The listing builds one solid part. Answer for the finished solid, in the listing's coordinates (mm). Give positions to 0.01 mm unless a question says otherwise; leave off trailing zeros. Order: outer loops, then holes, each group sorted by start corner. A loop starts at its lowest first (then second) coordinate and runs counter-clockwise, first axis right, second up. Notation, with made-up numbers: (-18, 13.25) - (11, 13.25) arc R26 cw to (11, 44.25) - close; hole circle Ø3 at (37.25, 82.5). An arc over 180 degrees is marked (long way). Answer in a Markdown table with one row per item.
Autodesk Inventor part; units mm, degrees
ref_plane "YZ Plane" through (0, 0, 0) normal (1, 0, 0) x (0, 1, 0)
ref_plane "XZ Plane" through (0, 0, 0) normal (0, 1, 0) x (-1, 0, 0)
ref_plane "XY Plane" through (0, 0, 0) normal (0, 0, 1) x (1, 0, 0)
sketch "Sketch1" plane through (0, 0, 0) normal (0, 0, 1) x (1, 0, 0)
  line L0 (250.9966, 205.3522) -> (187.4463, 315.4245)
  line L1 (187.4463, 315.4245) -> (-0.0002, 315.4245)
  line L2 (157.2736, 43.0193) -> (250.9966, 205.3522)
  line L3 (-63.5502, -119.3142) -> (63.5503, -119.3142)
  line L4 (63.5503, -119.3142) -> (157.2736, 43.0193)
  line L5 (-157.2732, 43.0188) -> (-63.5502, -119.3142)
  line L6 (-187.4461, 315.4245) -> (-250.9964, 205.3523)
  line L7 (-250.9964, 205.3523) -> (-157.2732, 43.0188)
  line L8 (-0.0002, 315.4245) -> (-187.4461, 315.4245)
extrude "Extrusion1" add sketch "Sketch1" along normal blind 3
properties part number "glass" material "Glass"
Item 1: Find section B-B on y = -8.5. Write down the section's boundary in (x, z), then the cut area to 3 significant figures.
Answer block:
| item | result |
|---|---|
| outline | (-127.53, 0) - (127.53, 0) - (127.53, 3) - (-127.53, 3) - close |
| area | 765 mm² |
Item 2: Consider line 1 (X direction, y = 151.5, z = 1.55) (3 decimals); line 2 (Y direction, x = 202.5, z = 0.5); line 3 (X direction, y = -59, z = 2.2). Determine where each line is inside the solid, lowest interval first.
Answer block:
| item | result |
|---|---|
| line 1 | -219.905 to 219.905 |
| line 2 | 121.35 to 289.35 |
| line 3 | -98.37 to 98.37 |
Item 3: Find section C-C on x = -127.5. Write down the section's boundary in (y, z).
Answer block:
| item | result |
|---|---|
| outline | (-8.55, 0) - (315.42, 0) - (315.42, 3) - (-8.55, 3) - close |
Item 4: Find section A-A on z = 2.05. Write down the section's boundary in (x, y), then the cut area to 3 significant figures.
Answer block:
| item | result |
|---|---|
| outline | (-251, 205.35) - (-157.27, 43.02) - (-63.55, -119.31) - (63.55, -119.31) - (157.27, 43.02) - (251, 205.35) - (187.45, 315.42) - (-187.45, 315.42) - close |
| area | 150,000 mm² |
